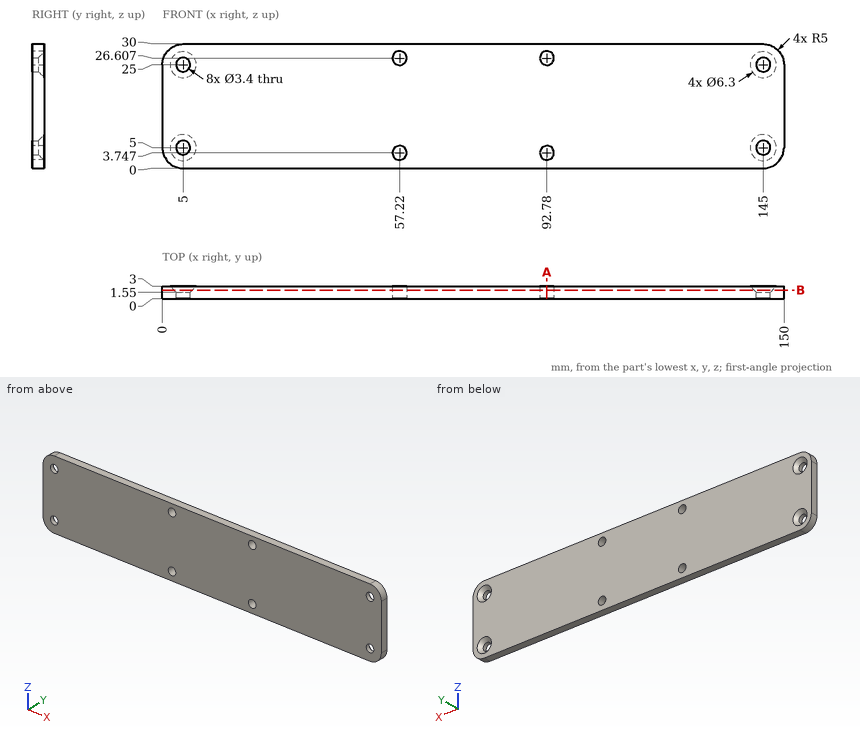
Drawing for the job (mm, zero at the part's lowest x, y, z). Round coordinates to 2 decimals unless told otherwise and drop trailing zeros. Write each loop counter-clockwise with the first axis right and the second up, starting at its lowest first coordinate (ties: lowest second). Pieces come first, ordered by that corner, then holes. Notation, with made-up numbers: M 16,10.5 L 29,10.5 A35 cw 29,42.5 Z; hole C -15,29 d4. An arc over 180 degrees is marked long. Answer as a JSON object with one key per item and string values. Group by question number.
(1) Cut at A-A (x = 92.78). Give the cut face in (y, z).
(2) Drill centre lines: L1, parallel to Z at x = 57, y = 2; L2, parallel to Z at x = 57.22, y = 1.2; L3, parallel to X at y = 1, z = 5. Where is each one in solid material? Low to high.
(3) Cut at B-B (y = 2.1). Give the number of separate pieces and of enclosed holes in the cut face, and give its area (3 significant figures).
(4) Flat gauge pins, fed straight in: pin 1 (4.5 mm diameter, centred on x = 145, z = 5, fed in from +Y); pin 2 (4.5 mm diameter, centred on x = 57.22, z = 3.75, fed in from +Y). Where does each tip first touch, or does it go through?
Responses:
{
 "1": {"outline": "M 0,0 L 3,0 L 3,2.05 L 0,2.05 Z; M 0,5.45 L 3,5.45 L 3,24.91 L 0,24.91 Z; M 0,28.31 L 3,28.31 L 3,30 L 0,30 Z"},
 "2": {"L1": "z = 0 to 2.06, 5.43 to 24.92, 28.29 to 30", "L2": "z = 0 to 2.05, 5.45 to 24.91, 28.31 to 30", "L3": "x = 0 to 3.3, 6.7 to 56.07, 58.37 to 91.63, 93.93 to 143.3, 146.7 to 150"},
 "3": {"separate pieces": "1", "enclosed holes": "8", "area": "4,380 mm2"},
 "4": {"pin 1": "stops at y = 2.1", "pin 2": "stops at y = 3"}
}
